Geometry check sheet. Reference: drawing and pictorial views, mm from the part's lowest x, y, z. A direction names the side the tool comes from. Coordinates: 2 decimals unless noted, no trailing zeros. Loops run counter-clockwise (first coordinate to the right, second up) from the corner with the lowest first, then second, coordinate; pieces in that order, holes last. Notation, with made-up numbers: (88.25, 30.25) - (99.25, 30.25) arc R24 ccw to (99.25, 55.25) - close; hole circle Ø11 at (-29.75, 83.5). An arc over 180 degrees is marked (long way). One line per item, written item: value.
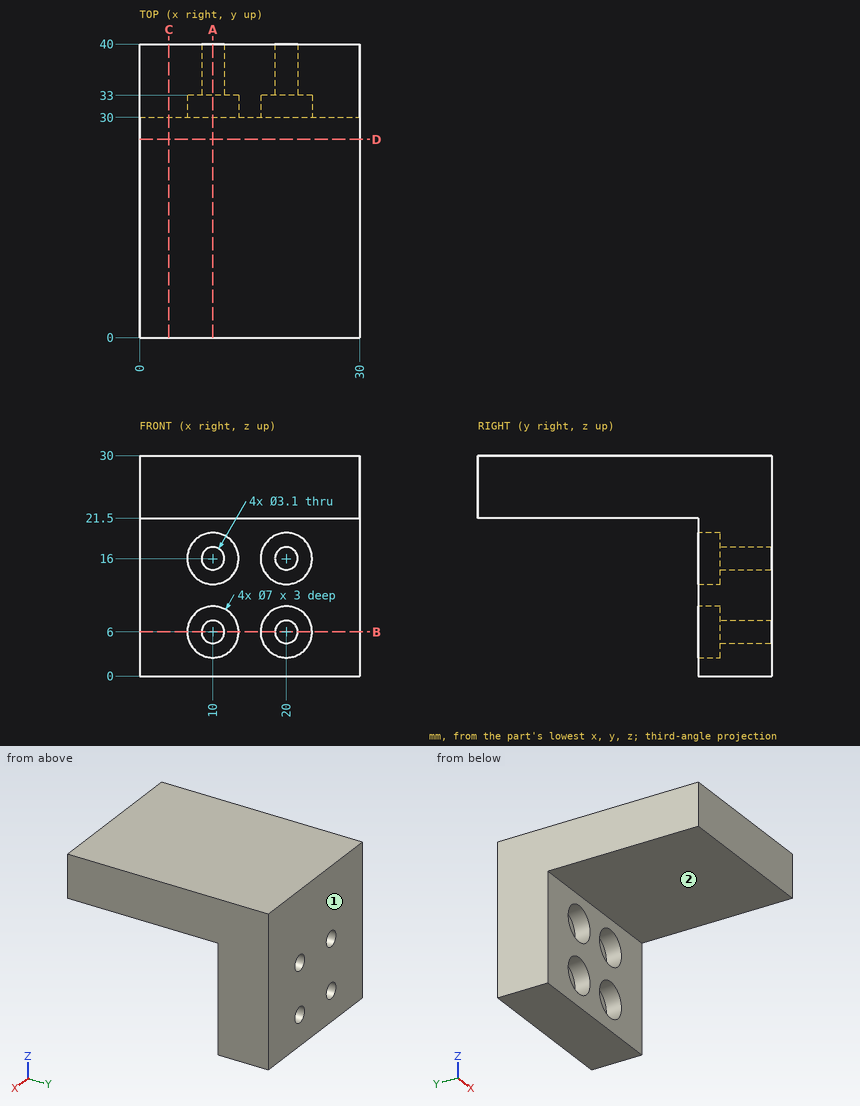
(1) Access from +Z, -Z, +X, -X, +Y, -Y to the whole of each face (thin tool, end or side, straight path). Record for the marked faces 1 and 2.
Reply:
face 1: +Z, -Z, +X, -X, +Y
face 2: -Z, +X, -X, -Y
(2) Cross-section at A-A on x = 10. Record the cut outline in (y, z), and give its area (3 significant figures).
Reply:
outline: (0, 21.5) - (30, 21.5) - (30, 19.5) - (33, 19.5) - (33, 17.55) - (40, 17.55) - (40, 30) - (0, 30) - close; (30, 0) - (40, 0) - (40, 4.45) - (33, 4.45) - (33, 2.5) - (30, 2.5) - close; (30, 9.5) - (33, 9.5) - (33, 7.55) - (40, 7.55) - (40, 14.45) - (33, 14.45) - (33, 12.5) - (30, 12.5) - close
area: 470 mm2
(3) Go/stop test with flat-tipped pins: pin 1 Ø1.9 at (x, z) = (10, 16) entering from +Y; pin 2 Ø4 at (x, z) = (10, 16) entering from -Y; pin 3 Ø11 at (x, z) = (20, 7.5) entering from -Y; pin 4 Ø15 at (x, y) = (11.5, 16.5) entering from -Z. Record where each tip stops, or that it passes through.
Reply:
pin 1: through
pin 2: y = 33
pin 3: y = 30
pin 4: z = 21.5
(4) Cross-section at C-C on x = 4. Record the cut outline in (y, z).
Reply:
outline: (0, 21.5) - (30, 21.5) - (30, 0) - (40, 0) - (40, 30) - (0, 30) - close
(5) Material ranges on probe 1 along X at (y, z) = (38.5, 6); probe 2 along X at (y, z) = (31.4, 6); probe 3 along Z at (x, y) = (9.75, 31.5), recorded low to high. Write a range as from..to.
Reply:
probe 1: 0..8.45, 11.55..18.45, 21.55..30
probe 2: 0..6.5, 13.5..16.5, 23.5..30
probe 3: 0..2.51, 9.49..12.51, 19.49..30
(6) Cross-section at D-D on y = 27. Record the cut outline in (x, z), and give its area (3 significant figures).
Reply:
outline: (0, 21.5) - (30, 21.5) - (30, 30) - (0, 30) - close
area: 255 mm2
(7) Cross-section at B-B on z = 6. Record the cut outline in (x, y), and give its area (3 significant figures).
Reply:
outline: (0, 30) - (6.5, 30) - (6.5, 33) - (8.45, 33) - (8.45, 40) - (0, 40) - close; (11.55, 33) - (13.5, 33) - (13.5, 30) - (16.5, 30) - (16.5, 33) - (18.45, 33) - (18.45, 40) - (11.55, 40) - close; (21.55, 33) - (23.5, 33) - (23.5, 30) - (30, 30) - (30, 40) - (21.55, 40) - close
area: 215 mm2
